The model under review builds one solid part; all positions refer to its coordinate system, in mm. A direction names the side the tool comes from. Coordinates: 2 decimals unless noted, no trailing zeros. Write each loop counter-clockwise with the first axis right and the second up, starting at its lowest first coordinate (ties: lowest second). Pieces come first, ordered by that corner, then holes.
```python
from build123d import *

# Parameters (mm, degrees)
EXTRUDE_1_DEPTH                = 2
HOLE_WIZARD_M3_5_1_D           = 2.9
HOLE_WIZARD_M3_5_1_DEPTH       = 8.8
HOLE_WIZARD_M3_5_1_CSINK_D     = 3.55
HOLE_WIZARD_M3_5_1_CSINK_ANGLE = 90
HOLE_WIZARD_M3_5_1_TIP         = 0.871247898
SKETCH_4_R                     = 15
SKETCH_4_R_2                   = 10.25
EXTRUDE_2_DEPTH                = 50


with BuildPart() as part:
    # 草图1 → 凸台-拉伸1 (new body)
    with BuildSketch(Plane(origin=(0, 0, 0), x_dir=(1, 0, 0), z_dir=(0, 1, 0))):
        Polygon((0, -15), (0, 0), (0, 30), (-30, 30), (-57, 30), (-60, 30), (-60, 0), (-60, -15), align=None)
    extrude(amount=EXTRUDE_1_DEPTH)

    # M3.5 螺纹孔1
    with Locations(Plane(origin=(0, 2, 0), x_dir=(1, 0, 0), z_dir=(0, 1, 0))):
        with Locations((-57, 25), (-3, 25)):
            CounterSinkHole(HOLE_WIZARD_M3_5_1_D / 2, HOLE_WIZARD_M3_5_1_CSINK_D / 2, depth=HOLE_WIZARD_M3_5_1_DEPTH, counter_sink_angle=HOLE_WIZARD_M3_5_1_CSINK_ANGLE)
            with Locations((0, 0, -(HOLE_WIZARD_M3_5_1_DEPTH + HOLE_WIZARD_M3_5_1_TIP / 2))):  # 118° drill point
                Cone(0, HOLE_WIZARD_M3_5_1_D / 2, HOLE_WIZARD_M3_5_1_TIP, mode=Mode.SUBTRACT)

    # 草图4 → 凸台-拉伸2 (add)
    with BuildSketch(Plane(origin=(0, 2, 0), x_dir=(1, 0, 0), z_dir=(0, 1, 0))):
        with Locations(Location((-30, 2.5, 0), (0, 0, 270))):
            Circle(SKETCH_4_R)
        with Locations(Location((-30, 2.5, 0), (0, 0, 270))):
            Circle(SKETCH_4_R_2, mode=Mode.SUBTRACT)
    extrude(amount=EXTRUDE_2_DEPTH)


solid = part.part
```
Item 1: For pin 1 (5 mm diameter, centred on x = -40, y = 43.5, fed in from -Z); pin 2 (8 mm diameter, centred on x = -11, z = -18.5, fed in from -Y); pin 3 (6 mm diameter, centred on x = -20, y = 7, fed in from -Z); pin 4 (1.5 mm diameter, centred on y = 19, z = -6.5, fed in from +X), all flat-tipped, find the tip position at first contact; note any pin that passes through.
Solved:
pin 1: stops at z = -15.49
pin 2: stops at y = 0
pin 3: stops at z = -15.77
pin 4: stops at x = -15.36
Item 2: To check wall thickness, follow line 1 along X through (y, z) = (0.9, -25); line 2 along X through (y, z) = (18, -2); line 3 along Z through (x, y) = (-3, 1.3). State the ranges of each line that lie inside material, in increasing order.
Solved:
line 1: x = -60 to -58.45, -55.55 to -4.45, -1.55 to 0
line 2: x = -44.99 to -40.24, -19.76 to -15.01
line 3: z = -30 to -26.45, -23.55 to 15
Item 3: Take a section at D-D, the plane y = 27. Write out the cut boundary in (x, z).
Solved:
outline: circle Ø30 at (-30, -2.5); hole circle Ø20.5 at (-30, -2.5)
Item 4: Take a section at B-B, the plane x = -57. Write out the cut boundary in (y, z) (3 decimals).
Solved:
outline: (0, -30) - (2, -30) - (2, -26.775) - (1.675, -26.45) - (0, -26.45) - close; (0, -23.55) - (1.675, -23.55) - (2, -23.225) - (2, 15) - (0, 15) - close
Item 5: Mouldability with a two-part tool opening along Z and no side actions: class faces 1 (the face through (-40, 52, 1)), 2 (the face through (-30, 1, 15)), 3 (the face through (-40.006, 26.65, -4.722)) as pulls with the +Z half, pulls with the -Z half, needs draft (parallel to the pull), parting line crosses it, or undercut.
Solved:
face 1: needs draft
face 2: pulls with the +Z half
face 3: undercut
Item 6: Machinability: for faces 4 (the face through (-30, 2, -3)), 5 (the face through (-55.55, 0.83, -25.06)), which of the approach directions +Z, -Z, +X, -X, +Y, -Y give a long, thin tool a straight path to every point of the face, cutting with its end or side? Answer none if there is none.
Solved:
face 4: +Y
face 5: +Y, -Y
Item 7: Take a section at C-C, the plane z = -2.5. Write out the cut boundary in (x, y), plus the area to 3 significant figures.
Solved:
outline: (-60, 0) - (0, 0) - (0, 2) - (-15, 2) - (-15, 52) - (-19.75, 52) - (-19.75, 2) - (-40.25, 2) - (-40.25, 52) - (-45, 52) - (-45, 2) - (-60, 2) - close
area: 595 mm2
Item 8: Take a section at A-A, the plane z = -25. Write out the cut boundary in (x, y) (3 decimals).
Solved:
outline: (-60, 0) - (-58.45, 0) - (-58.45, 1.675) - (-58.775, 2) - (-60, 2) - close; (-55.55, 0) - (-4.45, 0) - (-4.45, 1.675) - (-4.775, 2) - (-55.225, 2) - (-55.55, 1.675) - close; (-1.55, 0) - (0, 0) - (0, 2) - (-1.225, 2) - (-1.55, 1.675) - close
